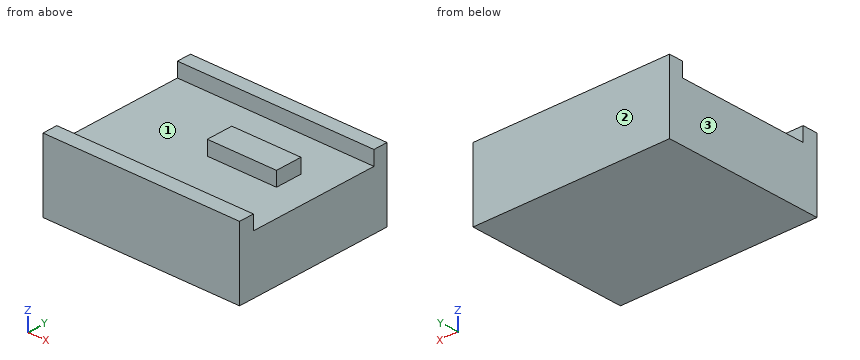
```python
from build123d import *

# Parameters (mm, degrees)
F0_W     = 69.85
F0_H     = 46.728912
F0_R     = 3.018536
F0_W_2   = 24.570362
F0_H_2   = 9.496521
F1_DEPTH = 20.32
F0_H_3   = 5.360574
F0_H_4   = 5.060514
F2_DEPTH = 25.4


with BuildPart() as f1:
    # F0 (on Top) → F1 (new body)
    with BuildSketch(Plane.XY):
        with Locations((-30.394862, 8.510193)):
            Rectangle(F0_W, F0_H)
        with Locations((-56.652177, -5.056264)):
            Circle(F0_R, mode=Mode.SUBTRACT)
        with BuildLine():
            ThreePointArc((-47.310162, -5.056264), (-50.471902, -8.218004), (-53.633642, -5.056264))
            ThreePointArc((-53.633642, -5.056264), (-50.471902, -1.894525), (-47.310162, -5.056264))
        make_face(mode=Mode.SUBTRACT)
        with Locations((-19.042942, 11.148115)):
            Rectangle(F0_W_2, F0_H_2, mode=Mode.SUBTRACT)
        with Locations((-56.652177, -5.056264)):
            Circle(F0_R)
        with BuildLine():
            ThreePointArc((-47.310162, -5.056264), (-50.471902, -1.894525), (-53.633642, -5.056264))
            ThreePointArc((-53.633642, -5.056264), (-50.471902, -8.218004), (-47.310162, -5.056264))
        make_face()
    extrude(amount=F1_DEPTH)

    # F0 (on Top) → F2 (join)
    with BuildSketch(Plane.XY):
        with Locations((-19.042942, 11.148115)):
            Rectangle(F0_W_2, F0_H_2)
        with Locations((-30.394862, -17.53455)):
            Rectangle(F0_W, F0_H_3)
        with Locations((-30.394862, 34.404906)):
            Rectangle(F0_W, F0_H_4)
    extrude(amount=F2_DEPTH)


solid = f1.part
```
Source: CAD feature listing. Evaluate the final solid. Frame: model axes, mm. Face numbers are marked on the shaded views. Coordinates: 2 decimals unless noted, no trailing zeros. Loops run counter-clockwise (first coordinate to the right, second up) from the corner with the lowest first, then second, coordinate; pieces in that order, holes last. Notation, with made-up numbers: M -21.5,-35.5 L 1.5,-35.5 A31 ccw 1.5,2.5 Z; hole C 2,29 d10. An arc over 180 degrees is marked long. Use a Markdown table: item, result. Add a question column.
Q1. Draft query along Y for the marked faces 1, 2 and 3. Return one class per face: pulls with the +Y half, pulls with the -Y half, needs draft (parallel to the pull), parting line crosses it, or undercut.
Q2. Section query C-C, the plane x = -4.5. Return loops of the section in (y, z).
Q3. Section query D-D, the plane y = -8.5. Return loops of the section in (x, z), and give its area (3 significant figures).
Q4. First-contact query: pin 1 (4 mm diameter, centred on y = 9, z = 24, fed in from +X); pin 2 (5.5 mm diameter, centred on y = 13.5, z = 24, fed in from -X); pin 3 (1 mm diameter, centred on x = -12.5, y = 27.5, fed in from +Z). Flat tips, straight axial feed; report the tip coordinate or a pass-through.
Q5. Material intervals for L1, parallel to Z at x = -60, y = 0; L2, parallel to Y at x = -54, z = 24.25, sorted ascending.
Q6. Section query A-A, the plane x = -28. Return loops of the section in (y, z), and give its area (3 significant figures).
Q7. Section query B-B, the plane y = 12. Return loops of the section in (x, z), and give its area (3 significant figures).
Result:
| question | item | result |
|---|---|---|
| 1 | face 1 | undercut |
| 1 | face 2 | pulls with the +Y half |
| 1 | face 3 | needs draft |
| 2 | outline | M -20.21,0 L 36.94,0 L 36.94,25.4 L 31.87,25.4 L 31.87,20.32 L -14.85,20.32 L -14.85,25.4 L -20.21,25.4 Z |
| 3 | outline | M -65.32,0 L 4.53,0 L 4.53,20.32 L -65.32,20.32 Z |
| 3 | area | 1,420 mm2 |
| 4 | pin 1 | stops at x = -6.76 |
| 4 | pin 2 | stops at x = -31.33 |
| 4 | pin 3 | stops at z = 20.32 |
| 5 | L1 | z = 0 to 20.32 |
| 5 | L2 | y = -20.21 to -14.85, 31.87 to 36.94 |
| 6 | outline | M -20.21,0 L 36.94,0 L 36.94,25.4 L 31.87,25.4 L 31.87,20.32 L 15.9,20.32 L 15.9,25.4 L 6.4,25.4 L 6.4,20.32 L -14.85,20.32 L -14.85,25.4 L -20.21,25.4 Z |
| 6 | area | 1,260 mm2 |
| 7 | outline | M -65.32,0 L 4.53,0 L 4.53,20.32 L -6.76,20.32 L -6.76,25.4 L -31.33,25.4 L -31.33,20.32 L -65.32,20.32 Z |
| 7 | area | 1,540 mm2 |
